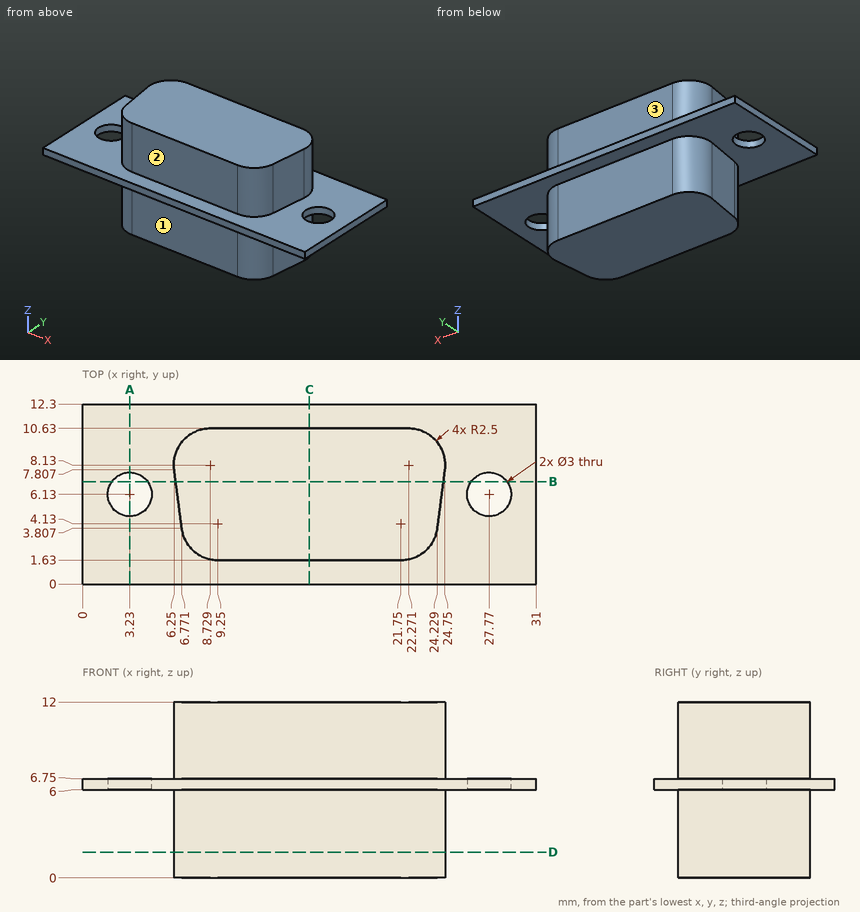
Source: three-view drawing plus pictorial views. Frame: mm from the lowest corner of the part. A direction names the side the tool comes from. Give positions to 0.01 mm unless a question says otherwise; leave off trailing zeros. Order: outer loops, then holes, each group sorted by start corner. A loop starts at its lowest first (then second) coordinate and runs counter-clockwise, first axis right, second up. Notation, with made-up numbers: M 82,12 L 137,12 A22 ccw 137,47 Z; hole C -23,12.25 d4. An arc over 180 degrees is marked long. Return JSON: item names as keys, results as strings.
1) Section query B-B on y = 7. Output: boundary loops of the cut face in (x, z) (3 decimals).
Taken from the geometry:
{"outline": "M 0,6 L 2.008,6 L 2.008,6.75 L 0,6.75 Z; M 4.452,6 L 6.355,6 L 6.355,0 L 24.645,0 L 24.645,6 L 26.548,6 L 26.548,6.75 L 24.645,6.75 L 24.645,12 L 6.355,12 L 6.355,6.75 L 4.452,6.75 Z; M 28.992,6 L 31,6 L 31,6.75 L 28.992,6.75 Z"}
2) Line query: L1, parallel to Y at x = 27.77, z = 6.55; L2, parallel to X at y = 6.13, z = 6.3; L3, parallel to Z at x = 28.5, y = 3.75. Output: solid intervals per line, ascending. Write a range as [from, to].
Taken from the geometry:
{"L1": "y = [0, 4.63], [7.63, 12.3]", "L2": "x = [0, 1.73], [4.73, 26.27], [29.27, 31]", "L3": "z = [6, 6.75]"}
3) Section query C-C on x = 15.5. Output: boundary loops of the cut face in (y, z), and give its area (3 significant figures).
Taken from the geometry:
{"outline": "M 0,6 L 1.63,6 L 1.63,0 L 10.63,0 L 10.63,6 L 12.3,6 L 12.3,6.75 L 10.63,6.75 L 10.63,12 L 1.63,12 L 1.63,6.75 L 0,6.75 Z", "area": "110 mm2"}
4) Section query D-D on z = 1.75. Output: boundary loops of the cut face in (x, y).
Taken from the geometry:
{"outline": "M 6.25,7.81 L 6.77,3.81 A2.5 ccw 9.25,1.63 L 21.75,1.63 A2.5 ccw 24.23,3.81 L 24.75,7.81 A2.5 ccw 22.27,10.63 L 8.73,10.63 A2.5 ccw Z"}
5) Access query for the marked faces 1, 2 and 3. Directions: +Z, -Z, +X, -X, +Y, -Y. A direction counts if a zero-diameter tool reaches every point of the face in a straight line with its end or side. Return the directions, or none.
Taken from the geometry:
{"face 1": "-Z, +X, -X, -Y", "face 2": "+Z, +X, -X, -Y", "face 3": "+Z, +X, -X, +Y"}
6) Section query A-A on x = 3.23. Output: boundary loops of the cut face in (y, z).
Taken from the geometry:
{"outline": "M 0,6 L 4.63,6 L 4.63,6.75 L 0,6.75 Z; M 7.63,6 L 12.3,6 L 12.3,6.75 L 7.63,6.75 Z"}
7) Contact query for flat-ended pins moving along their axis: pin 1 (1.5 mm diameter, centred on x = 24.5, z = 8, fed in from -Y); pin 2 (1 mm diameter, centred on x = 14.5, z = 8, fed in from +Y); pin 3 (6 mm diameter, centred on x = 16.5, z = 9.5, fed in from -Y); pin 4 (3 mm diameter, centred on x = 18, z = 2.5, fed in from -Y). Output: stop coordinate, or through.
Taken from the geometry:
{"pin 1": "stops at y = 2.63", "pin 2": "stops at y = 10.63", "pin 3": "stops at y = 0", "pin 4": "stops at y = 1.63"}
